Model file for the job. Use its own axes, mm. A direction names the side the tool comes from. Round coordinates to 2 decimals unless told otherwise and drop trailing zeros. Order: outer loops, then holes, each group sorted by start corner. A loop starts at its lowest first (then second) coordinate and runs counter-clockwise, first axis right, second up. Notation, with made-up numbers: (77, 52) -> (95, 52) arc R12 cw to (95, 65) -> close; hole circle Ø7 at (52.5, -16). An arc over 180 degrees is marked (long way). Use CSV: the item, a comma, the result in double quotes.
```python
from build123d import *

# Parameters (mm, degrees)
F0_W      = 750
F0_H      = 750
F1_DEPTH  = 600
F3_DEPTH  = 25
F4_W      = 100
F4_H      = 500
F5_DEPTH  = 100
F6_W      = 400
F6_H      = 200
F7_DEPTH  = 150
F10_DEPTH = 100
F11_DEPTH = 100
F12_R     = 150
F14_DEPTH = 200
F13_R     = 150
F15_DEPTH = 200
F17_DEPTH = 375
F18_T     = -3
F21_DEPTH = 100
F22_DEPTH = 100
F23_R     = 50
F24_DEPTH = 850
F25_W     = 300
F25_H     = 100
F26_DEPTH = 100
F30_W     = 100
F30_H     = 200
F31_DEPTH = 100


with BuildPart() as f1:
    # F0 (on Front) → F1 (new body, symmetric)
    with BuildSketch(Plane.XZ):
        with Locations((0, 525)):
            Rectangle(F0_W, F0_H)
    extrude(amount=F1_DEPTH, both=True)

    # F2 (on face) → F3 (join)
    with BuildSketch(Plane.XY.offset(900)):
        Polygon((-800, -450), (-375, -600), (375, -600), (800, -450), (800, 200), (375, 600), (-375, 600), (-800, 200), align=None)
    extrude(amount=F3_DEPTH)

    # F4 (on face) → F5 (join)
    with BuildSketch(Plane(origin=(-375, 0, 0), x_dir=(0, -1, 0), z_dir=(-1, 0, 0))):
        with Locations((650, 900)):
            Rectangle(F4_W, F4_H)
    extrude(amount=-F5_DEPTH)

    # F6 (on face) → F7 (join)
    with BuildSketch(Plane(origin=(0, -600, 0), x_dir=(-1, 0, 0), z_dir=(0, 1, 0))):
        with Locations((325, 1250)):
            Rectangle(F6_W, F6_H)
    extrude(amount=-F7_DEPTH)

    # F8 (on face) → F10 (join)
    with BuildSketch(Plane(origin=(-375, 0, 0), x_dir=(0, -1, 0), z_dir=(-1, 0, 0))):
        Polygon((50, 300), (-50, 300), (-750, 176.5711135041), (-750, 0), (-650, 0), (-650, 92.6611503863), (-50, 198.4573388114), (-50, 0), (50, 0), (50, 198.4573388114), (650, 92.6611503863), (650, 0), (750, 0), (750, 176.5711135041), align=None)
    extrude(amount=F10_DEPTH)

    # F9 (on face) → F11 (join)
    with BuildSketch(Plane.YZ.offset(375)):
        Polygon((-750, 176.5711135041), (-750, 0), (-650, 0), (-650, 92.6611503863), (-50, 198.4573388114), (-50, 0), (50, 0), (50, 198.4573388114), (650, 92.6611503863), (650, 0), (750, 0), (750, 176.5711135041), (50, 300), (-50, 300), align=None)
    extrude(amount=F11_DEPTH)

    # F12 (on face) → F14 (join)
    with BuildSketch(Plane.YZ.offset(475)):
        with Locations((-700, 0)):
            Circle(F12_R)
        Circle(F12_R)
        with Locations((700, 0)):
            Circle(F12_R)
    extrude(amount=F14_DEPTH)

    # F13 (on face) → F15 (join)
    with BuildSketch(Plane(origin=(-475, 0, 0), x_dir=(0, -1, 0), z_dir=(-1, 0, 0))):
        with Locations((-700, 0)):
            Circle(F13_R)
        Circle(F13_R)
        with Locations((700, 0)):
            Circle(F13_R)
    extrude(amount=F15_DEPTH)



with BuildPart() as f17:
    # F16 (on Right) → F17 (new body, symmetric)
    with BuildSketch(Plane.YZ):
        with BuildLine():
            Line((869.1369255612, 1180.2128462175), (630.8630744388, 1619.7871537825))
            ThreePointArc((630.8630744388, 1619.7871537825), (530.2128462175, 1280.8630744388), (869.1369255612, 1180.2128462175))
        make_face()
    extrude(amount=F17_DEPTH, both=True)

    # F18
    f18_openings = [f17.faces().sort_by_distance(p)[0] for p in [
        (0, 750, 1400),
    ]]
    offset(amount=F18_T, openings=f18_openings)


with BuildPart() as f1_1:
    add(f1.part)

    add(f17.part)  # F21 merges F17
    # F19 (on face) → F21 (join)
    with BuildSketch(Plane(origin=(-375, 0, 0), x_dir=(0, -1, 0), z_dir=(-1, 0, 0))):
        Polygon((-468.7665680933, 543.607708595), (-701.7037086855, 1412.9409522551), (-798.2962913145, 1387.0590477449), (-565.3591507222, 517.7258040847), align=None)
    extrude(amount=F21_DEPTH)

    # F20 (on face) → F22 (join)
    with BuildSketch(Plane.YZ.offset(375)):
        Polygon((701.7037086855, 1412.9409522551), (468.7665680933, 543.607708595), (565.3591507222, 517.7258040847), (798.2962913145, 1387.0590477449), align=None)
    extrude(amount=F22_DEPTH)



with BuildPart() as f24:
    # F23 (on face) → F24 (new body)
    with BuildSketch(Plane.XZ.offset(600)):
        with Locations((450, 820)):
            Circle(F23_R)
    extrude(amount=-F24_DEPTH)


with BuildPart() as f24b:
    # F23 (on face) → F24, piece 2 (new body)
    with BuildSketch(Plane.XZ.offset(600)):
        with Locations((450, 700)):
            Circle(F23_R)
    extrude(amount=-F24_DEPTH)


with BuildPart() as f24c:
    # F23 (on face) → F24, piece 3 (new body)
    with BuildSketch(Plane.XZ.offset(600)):
        with Locations((450, 520)):
            Circle(F23_R)
    extrude(amount=-F24_DEPTH)


with BuildPart() as f24d:
    # F23 (on face) → F24, piece 4 (new body)
    with BuildSketch(Plane.XZ.offset(600)):
        with Locations((450, 400)):
            Circle(F23_R)
    extrude(amount=-F24_DEPTH)


with BuildPart() as f24e:
    # F23 (on face) → F24, piece 5 (new body)
    with BuildSketch(Plane.XZ.offset(600)):
        with Locations((-450, 520)):
            Circle(F23_R)
    extrude(amount=-F24_DEPTH)


with BuildPart() as f24f:
    # F23 (on face) → F24, piece 6 (new body)
    with BuildSketch(Plane.XZ.offset(600)):
        with Locations((-450, 400)):
            Circle(F23_R)
    extrude(amount=-F24_DEPTH)


with BuildPart() as f1_2:
    add(f1_1.part)

    add(f24b.part)  # F26 merges F24b

    add(f24d.part)  # F26 merges F24d

    add(f24f.part)  # F26 merges F24f
    # F25 (on face) → F26 (join)
    with BuildSketch(Plane.XZ.offset(600)):
        with Locations((-400, 400)):
            Rectangle(F25_W, F25_H)
        with Locations((400, 400)):
            Rectangle(F25_W, F25_H)
        with Locations((400, 700)):
            Rectangle(F25_W, F25_H)
    extrude(amount=F26_DEPTH)

    # F27: union 

    # F28: union 

    # F29: union 


    add(f24.part)  # F31 merges F24

    add(f24c.part)  # F31 merges F24c

    add(f24e.part)  # F31 merges F24e
    # F30 (on face) → F31 (join)
    with BuildSketch(Plane(origin=(0, 250, 0), x_dir=(-1, 0, 0), z_dir=(0, 1, 0))):
        with Locations((-450, 450)):
            Rectangle(F30_W, F30_H)
        with Locations((450, 450)):
            Rectangle(F30_W, F30_H)
        with Locations((-450, 750)):
            Rectangle(F30_W, F30_H)
    extrude(amount=F31_DEPTH)


solid = f1_2.part
```
Q1. Cut at A-A (y = 0). State how many separate pieces and enclosed holes the cut face has, plus the area to 3 significant figures.
From the geometry:
separate pieces,"7"
enclosed holes,"0"
area,"830,000 mm²"
Q2. Cut at C-C (y = 278.5). Give the cut face in (x, z).
From the geometry:
outline,"(-716.59, 900) -> (-375, 900) -> (-375, 259.71) -> (-475, 259.71) -> (-475, 158.17) -> (-375, 158.17) -> (-375, 150) -> (375, 150) -> (375, 158.17) -> (475, 158.17) -> (475, 259.71) -> (375, 259.71) -> (375, 900) -> (716.59, 900) -> (716.59, 925) -> (-716.59, 925) -> close; (-500, 350) -> (-400, 350) -> (-400, 550) -> (-500, 550) -> close; (400, 350) -> (500, 350) -> (500, 550) -> (400, 550) -> close; (400, 650) -> (500, 650) -> (500, 850) -> (400, 850) -> close"
Q3. Probe line 1 along X through (y, z) = (-615.5, -27); line 2 along X through (y, z) = (-256.5, 425); line 3 along Z through (x, y) = (-309, -35). List the from-to ranges inside material, lowest first.
From the geometry:
line 1,"x = -675 to -475, 475 to 675"
line 2,"x = -493.3 to -406.7, -375 to 375, 406.7 to 493.3"
line 3,"z = 150 to 925"
Q4. Cut at B-B (x = 54). Give the cut face in (y, z), plus the area to 3 significant figures.
From the geometry:
outline,"(-600, 150) -> (600, 150) -> (600, 925) -> (-600, 925) -> close; (630.86, 1619.79) arc R250 ccw to (869.14, 1180.21) -> (867.71, 1182.85) arc R247 cw to (632.29, 1617.15) -> close"
area,"932,000 mm²"
Q5. Cut at D-D (z = 1508). Give the cut face in (x, y).
From the geometry:
outline,"(-375, 524.53) -> (375, 524.53) -> (375, 691.46) -> (372, 691.46) -> (372, 527.86) -> (-372, 527.86) -> (-372, 691.46) -> (-375, 691.46) -> close"
Q6. Which spindle directions (+Z, -Z, +X, -X, +Y, -Y) get a long thin tool onto all of the face, cutting with end or side? Do faces 4 (the flat face through (-424, -1, 300)), 5 (the flat face through (450, 250, 756)), 6 (the flat face through (-424.3, 683.46, 958.48)), 7 (the flat face through (-424, 701, 0)), 8 (the flat face through (451, 299, 650)). Say none if no direction does.
From the geometry:
face 4,"-X, +Y, -Y"
face 5,"none"
face 6,"-X, +Y"
face 7,"-Z, +Y, -Y"
face 8,"+X, -Y"
Q7. Pin check, flat tips, straight feed: pin 1 (3 mm diameter, centred on x = 487, y = 439.5, fed in from -Z); pin 2 (3 mm diameter, centred on y = 345.5, z = 277, fed in from -X); pin 3 (4 mm diameter, centred on x = -495.5, y = -406, fed in from -Z). Stop position of each tip, or through.
From the geometry:
pin 1,"stops at z = 900"
pin 2,"stops at x = -375"
pin 3,"stops at z = 375.35"
Q8. Mould opens along Y. For faces 1 (the flat face through (-451, -600, 521)), 2 (the cylindrical face through (-573.6, 561.438, -57.451)), 3 (the flat face through (398, -649, 350)) say: +Y half, -Y half, draft (parallel to the pull), parting line (faces both ways), or undercut.
From the geometry:
face 1,"-Y half"
face 2,"undercut"
face 3,"draft"
